from build123d import *

# Parameters (mm, degrees)
F0_W     = 90
F0_H     = 60
F1_DEPTH = 3
F2_R     = 4.5
F3_DEPTH = 25
F5_DEPTH = 0.2


with BuildPart() as f1:
    # F0 (on Front) → F1 (new body)
    with BuildSketch(Plane.XZ):
        with Locations((45, 30)):
            Rectangle(F0_W, F0_H)
    extrude(amount=F1_DEPTH)

    # F2 (on face) → F3 (cut)
    with BuildSketch(Plane.XZ.offset(3)):
        with Locations((75, 45)):
            Circle(F2_R)
    extrude(amount=-F3_DEPTH, mode=Mode.SUBTRACT)

    # F4 (on face) → F5 (join)
    with BuildSketch(Plane.XZ.offset(3)):
        with BuildLine():
            ThreePointArc((14.332417, 27.872751), (15.485688, 34.293498), (11.041055, 29.518432))
            ThreePointArc((11.041055, 29.518432), (9.831879, 22.985878), (14.332417, 27.872751))
        make_face()
        with BuildLine():
            ThreePointArc((11.041055, 44.518432), (9.831879, 37.985878), (14.332417, 42.872751))
            ThreePointArc((14.332417, 42.872751), (15.485688, 49.293498), (11.041055, 44.518432))
        make_face()
        with BuildLine():
            ThreePointArc((11.041055, 59.518432), (9.831879, 52.985878), (14.332417, 57.872751))
            ThreePointArc((14.332417, 57.872751), (15.485688, 64.293498), (11.041055, 59.518432))
        make_face()
        with BuildLine():
            ThreePointArc((26.041055, 29.518432), (24.831879, 22.985878), (29.332417, 27.872751))
            ThreePointArc((29.332417, 27.872751), (30.485688, 34.293498), (26.041055, 29.518432))
        make_face()
        with BuildLine():
            ThreePointArc((26.041055, 44.518432), (24.831879, 37.985878), (29.332417, 42.872751))
            ThreePointArc((29.332417, 42.872751), (30.485688, 49.293498), (26.041055, 44.518432))
        make_face()
        with BuildLine():
            ThreePointArc((26.041055, 59.518432), (24.831879, 52.985878), (29.332417, 57.872751))
            ThreePointArc((29.332417, 57.872751), (30.485688, 64.293498), (26.041055, 59.518432))
        make_face()
        with BuildLine():
            ThreePointArc((41.041055, 29.518432), (39.831879, 22.985878), (44.332417, 27.872751))
            ThreePointArc((44.332417, 27.872751), (45.485688, 34.293498), (41.041055, 29.518432))
        make_face()
        with BuildLine():
            ThreePointArc((41.041055, 44.518432), (39.831879, 37.985878), (44.332417, 42.872751))
            ThreePointArc((44.332417, 42.872751), (45.485688, 49.293498), (41.041055, 44.518432))
        make_face()
        with BuildLine():
            ThreePointArc((41.041055, 59.518432), (39.831879, 52.985878), (44.332417, 57.872751))
            ThreePointArc((44.332417, 57.872751), (45.485688, 64.293498), (41.041055, 59.518432))
        make_face()
        with BuildLine():
            ThreePointArc((56.041055, 29.518432), (54.831879, 22.985878), (59.332417, 27.872751))
            ThreePointArc((59.332417, 27.872751), (60.485688, 34.293498), (56.041055, 29.518432))
        make_face()
        with BuildLine():
            ThreePointArc((56.041055, 44.518432), (54.831879, 37.985878), (59.332417, 42.872751))
            ThreePointArc((59.332417, 42.872751), (60.485688, 49.293498), (56.041055, 44.518432))
        make_face()
        with BuildLine():
            ThreePointArc((56.041055, 59.518432), (54.831879, 52.985878), (59.332417, 57.872751))
            ThreePointArc((59.332417, 57.872751), (60.485688, 64.293498), (56.041055, 59.518432))
        make_face()
        with BuildLine():
            ThreePointArc((71.041055, 29.518432), (69.831879, 22.985878), (74.332417, 27.872751))
            ThreePointArc((74.332417, 27.872751), (75.485688, 34.293498), (71.041055, 29.518432))
        make_face()
        with BuildLine():
            ThreePointArc((71.041055, 44.518432), (69.831879, 37.985878), (74.332417, 42.872751))
            ThreePointArc((74.332417, 42.872751), (75.485688, 49.293498), (71.041055, 44.518432))
        make_face()
        with BuildLine():
            ThreePointArc((71.041055, 59.518432), (69.831879, 52.985878), (74.332417, 57.872751))
            ThreePointArc((74.332417, 57.872751), (75.485688, 64.293498), (71.041055, 59.518432))
        make_face()
    extrude(amount=F5_DEPTH)


solid = f1.part
Verification items for the finished model (mm, model axes). A direction names the side the tool comes from. Give positions to 0.01 mm unless a question says otherwise; leave off trailing zeros. Loops run counter-clockwise (first coordinate to the right, second up) from the corner with the lowest first, then second, coordinate; pieces in that order, holes last. Notation, with made-up numbers: (27.5, 81) - (66.5, 81) arc R9 cw to (66.5, 98) - close; hole circle Ø3 at (2.5, 73.5). An arc over 180 degrees is marked (long way). Write item = value, one per line. Start each with the question number.
Q1. Thickness scan on line 1 (Z direction, x = 75, y = -2.3); line 2 (X direction, y = -1.3, z = 45); line 3 (Y direction, x = 79.5, z = 43.5). Record the ranges inside material, lowest first.
Q2. Cross-section at C-C, the plane z = 32.5. Enter the section's corners in (x, y).
Q3. Depth check by flat-ended pin: P1, Ø1.5, axis at x = 61, y = -2, coming from the +Z side; P2, Ø1.4, axis at x = 28, z = 61.5, coming from the +Y side; P3, Ø3, axis at x = 72, z = 6.5, coming from the -Y side. Enter the tip coordinate at first touch or a pass-through.
Q4. Mould release check, pull along X, two halves, no side actions. Record for faces 1 (the face through (44.4, -3, 23.8)), 2 (the face through (28, -3.2, 59)): released by +X, released by -X, zero draft, split by the parting line, or undercut.
Q5. Cross-section at B-B, the plane z = 61. Enter the section's corners in (x, y), and give its area (3 significant figures).
Q6. Cross-section at D-D, the plane x = 35.5. Enter the section's corners in (y, z).
Q7. Cross-section at A-A, the plane y = -1.65. Enter the section's corners in (x, z), and give its area (3 significant figures).
Q8. Tool access check on faces 3 (the face through (29, -3, 62)), 4 (the face through (43, -3.2, 29)). Record the directions out of +Z, -Z, +X, -X, +Y, -Y that give a thin tool (end or side, any length) a straight path to the whole face; none if there is none.
Answer key:
q1.line_1 = 0 to 40.5, 49.5 to 60
q1.line_2 = 0 to 70.5, 79.5 to 90
q1.line_3 = -3 to 0
q2.outline = (0, -3) - (10.8, -3) - (10.8, -3.2) - (17.13, -3.2) - (17.13, -3) - (25.8, -3) - (25.8, -3.2) - (32.13, -3.2) - (32.13, -3) - (40.8, -3) - (40.8, -3.2) - (47.13, -3.2) - (47.13, -3) - (55.8, -3) - (55.8, -3.2) - (62.13, -3.2) - (62.13, -3) - (70.8, -3) - (70.8, -3.2) - (77.13, -3.2) - (77.13, -3) - (90, -3) - (90, 0) - (0, 0) - close
q3.P1 = 60
q3.P2 = -3
q3.P3 = -3
q4.face_1 = undercut
q4.face_2 = zero draft
q5.outline = (10.57, -3.2) - (17.36, -3.2) - (17.36, -3) - (10.57, -3) - close; (25.57, -3.2) - (32.36, -3.2) - (32.36, -3) - (25.57, -3) - close; (40.57, -3.2) - (47.36, -3.2) - (47.36, -3) - (40.57, -3) - close; (55.57, -3.2) - (62.36, -3.2) - (62.36, -3) - (55.57, -3) - close; (70.57, -3.2) - (77.36, -3.2) - (77.36, -3) - (70.57, -3) - close
q5.area = 6.78 mm^2
q6.outline = (-3, 0) - (0, 0) - (0, 60) - (-3, 60) - close
q7.outline = (0, 0) - (90, 0) - (90, 60) - (0, 60) - close; hole circle Ø9 at (75, 45)
q7.area = 5,340 mm^2
q8.face_3 = +Z, +X, -X, +Y
q8.face_4 = +Z, -Z, +X, -X, -Y
